The listing builds one solid part. Answer for the finished solid, in the listing's coordinates (mm). A direction names the side the tool comes from. Give positions to 0.01 mm unless a question says otherwise; leave off trailing zeros. Loops run counter-clockwise (first coordinate to the right, second up) from the corner with the lowest first, then second, coordinate; pieces in that order, holes last.
Item 1: Section A-A, the plane x = 0 is taken. Give the vertices of the cut face in (y, z), and give its area (3 significant figures).
Item 2: Section C-C, the plane z = -17 is taken. Give the vertices of the cut face in (x, y), and give its area (3 significant figures).
Item 3: A tool of negligible diameter and unlimited length cuts with its end or side. For faces 4 (the face through (6.466, 2.391, 18.798)), 5 (the face through (-0.521, 2.391, 15.034)), from which of +Z, -Z, +X, -X, +Y, -Y can it reach the whole face along a straight path? Write none if from no direction.
Item 4: Consider line 1 along Z through (x, y) = (0, 2.6); line 2 along Z through (x, y) = (-3, 1.8); line 3 along Z through (x, y) = (-1.5, 2.95). Determine where each line is inside the solid, lowest interval first.
Item 5: The mould has two halves that part along X. Classify faces 1 (the face through (0, 2, 2)), 2 (the face through (-0.1, 2.4, 25.5)), 3 (the face through (-6.465, 2.391, 18.781)): pulls with the +X half, pulls with the -X half, needs draft (parallel to the pull), parting line crosses it, or undercut.
Item 6: Section D-D, the plane z = 0 is taken. Give the vertices of the cut face in (x, y) (3 decimals), and give its area (3 significant figures).
Item 7: Section B-B, the plane y = 0.6 is taken. Give the vertices of the cut face in (x, z).
from build123d import *

# Parameters (mm, degrees)
SKETCH1_R           = 4
SKETCH1_R_2         = 1
SKETCH1_R_3         = 2
BOSS_EXTRUDE1_DEPTH = 4.85


with BuildPart() as part:
    # Sketch1 → Boss-Extrude1 (new body)
    with BuildSketch(Plane(origin=(0, 0, 0), x_dir=(1, 0, 0), z_dir=(0, 1, 0))):
        with BuildLine():
            Line((-3.666060556, 30.6), (-8.065333223, 20.52))
            ThreePointArc((-8.065333223, 20.52), (-8.667437744, 18.521684251), (-8.782021759, 16.437777778))
            ThreePointArc((-8.782021759, 16.437777778), (-8.64730319, 15.61122755), (-8.516431626, 14.784059485))
            ThreePointArc((-8.516431626, 14.784059485), (-6.724262557, -1.642204863), (-6.445963017, -18.163602496))
            ThreePointArc((-6.445963017, -18.163602496), (-6.465253257, -18.789475583), (-6.486720617, -19.415277778))
            ThreePointArc((-6.486720617, -19.415277778), (0, -25.5), (6.486720617, -19.415277778))
            ThreePointArc((6.486720617, -19.415277778), (6.465253257, -18.789475583), (6.445963017, -18.163602496))
            ThreePointArc((6.445963017, -18.163602496), (6.724262557, -1.642204863), (8.516431626, 14.784059485))
            ThreePointArc((8.516431626, 14.784059485), (8.64730319, 15.61122755), (8.782021759, 16.437777778))
            ThreePointArc((8.782021759, 16.437777778), (8.667437744, 18.521684251), (8.065333223, 20.52))
            Line((8.065333223, 20.52), (3.666060556, 30.6))
            ThreePointArc((3.666060556, 30.6), (0, 33), (-3.666060556, 30.6))
        make_face()
        with Locations((0, -19)):
            Circle(SKETCH1_R, mode=Mode.SUBTRACT)
        with Locations((0, -8)):
            Circle(SKETCH1_R_2, mode=Mode.SUBTRACT)
        Circle(SKETCH1_R_3, mode=Mode.SUBTRACT)
        with Locations((0, 17)):
            Circle(SKETCH1_R, mode=Mode.SUBTRACT)
        with Locations((0, 29)):
            Circle(SKETCH1_R_2, mode=Mode.SUBTRACT)
    extrude(amount=BOSS_EXTRUDE1_DEPTH)


solid = part.part
Worked answers:
1. outline: (0, -33) - (4.85, -33) - (4.85, -30) - (0, -30) - close; (0, -28) - (4.85, -28) - (4.85, -21) - (0, -21) - close; (0, -13) - (4.85, -13) - (4.85, -2) - (0, -2) - close; (0, 2) - (4.85, 2) - (4.85, 7) - (0, 7) - close; (0, 9) - (4.85, 9) - (4.85, 15) - (0, 15) - close; (0, 23) - (4.85, 23) - (4.85, 25.5) - (0, 25.5) - close
1. area: 167 mm2
2. outline: (-8.8, 0) - (-4, 0) - (-4, 4.85) - (-8.8, 4.85) - close; (4, 0) - (8.8, 0) - (8.8, 4.85) - (4, 4.85) - close
2. area: 46.6 mm2
3. face 4: +X, +Y, -Y
3. face 5: +Y, -Y
4. line 1: z = -33 to -30, -28 to -21, -13 to -2, 2 to 7, 9 to 15, 23 to 25.5
4. line 2: z = -31.65 to -19.65, -14.35 to 16.35, 21.65 to 24.77
4. line 3: z = -32.71 to -20.71, -13.29 to -1.32, 1.32 to 15.29, 22.71 to 25.32
5. face 1: undercut
5. face 2: parting line crosses it
5. face 3: pulls with the -X half
6. outline: (-6.835, 0) - (-2, 0) - (-2, 4.85) - (-6.835, 4.85) - close; (2, 0) - (6.835, 0) - (6.835, 4.85) - (2, 4.85) - close
6. area: 46.9 mm2
7. outline: (-8.78, -16.44) arc R8.8 ccw to (-8.07, -20.52) - (-3.67, -30.6) arc R4 ccw to (3.67, -30.6) - (8.07, -20.52) arc R8.8 ccw to (8.78, -16.44) arc R180 cw to (6.45, 18.16) arc R180 cw to (6.49, 19.42) arc R6.5 ccw to (-6.49, 19.42) arc R180 cw to (-6.45, 18.16) arc R180 cw to start; hole circle Ø8 at (0, -17); hole circle Ø8 at (0, 19); hole circle Ø4 at (0, 0); hole circle Ø2 at (0, -29); hole circle Ø2 at (0, 8)
